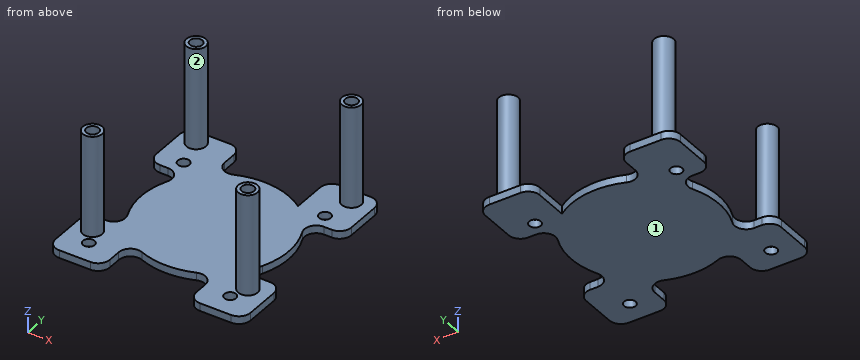
Autodesk Inventor part; units mm, degrees
ref_plane "Work Plane1" through (0, 0, 0) normal (0, 0, 1) x (1, 0, 0)
ref_plane "YZ Plane" through (0, 0, 0) normal (1, 0, 0) x (0, 1, 0)
ref_plane "XZ Plane" through (0, 0, 0) normal (0, 1, 0) x (-1, 0, 0)
ref_plane "Work Plane1" through (0, 0, 0) normal (0, 0, 1) x (1, 0, 0)
sketch "Sketch1" plane through (0, 0, 0) normal (0, 0, 1) x (1, 0, 0)
  circle A0 centre (22.2, -27.45) radius 1.5
  circle A1 centre (58.6, -27.45) radius 1.5
  circle A2 centre (22.2, 9.15) radius 1.5
  circle A3 centre (58.6, 9.15) radius 1.5
  line L0 (15.5, 16.5) -> (15.5, -25.3)
  line L1 (19.5, -29.3) -> (61, -29.3)
  line L2 (61, 20.5) -> (19.5, 20.5)
  line L3 (64.8607, 14) -> (64.8607, -18)
  line L4 (65.75, -18) -> (65.75, 14)
  line L5 (65.75, -33.3) -> (51.75, -33.3)
  line L6 (51.75, -33.3) -> (51.75, -21.8024)
  line L7 (55.4368, -18.3) -> (65.75, -18.3)
  line L8 (65.75, -18.3) -> (65.75, -33.3)
  line L9 (15.5, -33.3) -> (29.5, -33.3)
  line L10 (29.5, -33.3) -> (29.5, -21.8024)
  line L11 (25.8132, -18.3) -> (15.5, -18.3)
  line L12 (15.5, -18.3) -> (15.5, -33.3)
  line L13 (15.5, 20.5697) -> (29.5, 20.5697)
  line L14 (29.5, 20.5697) -> (29.5, 9.0024)
  line L15 (25.8695, 5.5697) -> (15.5, 5.5697)
  line L16 (15.5, 5.5697) -> (15.5, 20.5697)
  line L17 (51.75, 20.5697) -> (65.75, 20.5697)
  line L18 (65.75, 20.5697) -> (65.75, 5.5697)
  line L19 (65.75, 5.5697) -> (55.3805, 5.5697)
  line L20 (51.75, 9.0024) -> (51.75, 20.5697)
  arc A4 (51.75, 9.0024) -> (29.5, 9.0024) centre (40.625, -6.4) ccw
  arc A5 (25.8695, 5.5697) -> (25.8132, -18.3) centre (40.625, -6.4) ccw
  arc A6 (29.5, -21.8024) -> (51.75, -21.8024) centre (40.625, -6.4) ccw
  arc A7 (55.4368, -18.3) -> (55.3805, 5.5697) centre (40.625, -6.4) ccw
  line L21 (65.75, 20.5697) -> (65.75, 5.5697)
  line L22 (65.75, -18.3) -> (65.75, -33.3)
  line L23 (15.5, 20.5697) -> (29.5, 20.5697)
  line L24 (51.75, 20.5697) -> (65.75, 20.5697)
  line L25 (15.5, -33.3) -> (15.5, -18.3)
  line L26 (15.5, 5.5697) -> (15.5, 20.5697)
  point P0 (0, 0)
  point P1 (40.25, 20.5)
  dimension "d10" = 50.25
  dimension "d13" = 26.9
extrude "Extrusion1" add sketch "Sketch1" along normal blind 2 contours L16 L13 L14 A4 L20 L17 L18 L4 L19 A7 L7 L8 L5 L6 A6 L10 L9 L12 L0 L11 A5 L15
fillet "Fillet1" radius 3 7 edges at (55.3805, 5.5697, 1) (29.5, -21.8024, 1) (25.8132, -18.3, 1) (29.5, 9.0024, 1) (55.4368, -18.3, 1) (25.8695, 5.5697, 1) (51.75, -21.8024, 1)
fillet "Fillet2" radius 3 12 edges at (15.5, 20.5697, 1) (15.5, 5.5697, 1) (29.5, 20.5697, 1) (51.75, 20.5697, 1) (65.75, 20.5697, 1) (65.75, -18.3, 1) (51.75, -33.3, 1) (15.5, -18.3, 1) (15.5, -33.3, 1) (29.5, -33.3, 1) (65.75, -33.3, 1) (65.75, 5.5697, 1)
sketch "Sketch2" plane through (0, 0, 2) normal (0, 0, 1) x (1, 0, 0)
  circle A0 centre (60.25, -23.1) radius 1.6
  circle A1 centre (20.25, -23.1) radius 1.6
  circle A2 centre (20.25, 16.9) radius 1.6
  circle A3 centre (60.25, 16.9) radius 1.6
  circle A4 centre (20.25, -23.1) radius 2.5
  circle A5 centre (60.25, 16.9) radius 2.5
  circle A6 centre (20.25, 16.9) radius 2.5
  circle A7 centre (60.25, -23.1) radius 2.5
  point P0 (0, 0)
  dimension "d17" = 5
  dimension "d18" = 5
  dimension "d19" = 5
  dimension "d20" = 5
extrude "Extrusion2" add sketch "Sketch2" along normal blind 26
equation "\"d13\" = 0.5 * d11"
properties part number "soporteHBridge"
Verification items for the finished model (mm, model axes). Face numbers are marked on the shaded views. Coordinates: 2 decimals unless noted, no trailing zeros. Loops run counter-clockwise (first coordinate to the right, second up) from the corner with the lowest first, then second, coordinate; pieces in that order, holes last. Notation, with made-up numbers: (-26, 61) -> (24, 61) arc R12 ccw to (24, 74) -> close; hole circle Ø7 at (3, -40). An arc over 180 degrees is marked (long way). Answer as CSV lines item,"result".
1) Cross-section at B-B, the plane y = 16.9. Record the cut outline in (x, z).
Found:
outline,"(15.5, 0) -> (29.5, 0) -> (29.5, 2) -> (22.75, 2) -> (22.75, 28) -> (21.85, 28) -> (21.85, 2) -> (18.65, 2) -> (18.65, 28) -> (17.75, 28) -> (17.75, 2) -> (15.5, 2) -> close; (51.75, 0) -> (65.75, 0) -> (65.75, 2) -> (62.75, 2) -> (62.75, 28) -> (61.85, 28) -> (61.85, 2) -> (58.65, 2) -> (58.65, 28) -> (57.75, 28) -> (57.75, 2) -> (51.75, 2) -> close"
2) Cross-section at A-A, the plane z = 20.5. Record the cut outline in (x, y), then the cut area to 3 significant figures.
Found:
outline,"circle Ø5 at (20.25, -23.1); circle Ø5 at (20.25, 16.9); circle Ø5 at (60.25, -23.1); circle Ø5 at (60.25, 16.9); hole circle Ø3.2 at (20.25, -23.1); hole circle Ø3.2 at (20.25, 16.9); hole circle Ø3.2 at (60.25, -23.1); hole circle Ø3.2 at (60.25, 16.9)"
area,"46.4 mm2"
3) Depth check by flat-ended pin: pin 1 (3 mm diameter, centred on y = -21.5, z = 11, fed in from -X); pin 2 (3.5 mm diameter, centred on x = 60.25, y = 16.9, fed in from +Z); pin 3 (1.8 mm diameter, centred on x = 58.6, y = 9.15, fed in from -Z); pin 4 (12 mm diameter, centred on x = 22.5, y = 7.5, fed in from +Z). Enter the tip coordinate at first touch or a pass-through.
Found:
pin 1,"stops at x = 17.75"
pin 2,"stops at z = 28"
pin 3,"passes through"
pin 4,"stops at z = 2"
4) Cross-section at C-C, the plane x = 36.5. Record the cut outline in (y, z), then the cut area to 3 significant figures.
Found:
outline,"(-24.95, 0) -> (12.15, 0) -> (12.15, 2) -> (-24.95, 2) -> close"
area,"74.2 mm2"
5) Release check for a two-part mould opening along Y. For the marked faces 1 and 2 record: +Y half, -Y half, draft (parallel to the pull), parting line (faces both ways), or undercut.
Found:
face 1,"draft"
face 2,"undercut"
6) Cross-section at D-D, the plane y = -7.5. Record the cut outline in (x, z).
Found:
outline,"(21.66, 0) -> (59.59, 0) -> (59.59, 2) -> (21.66, 2) -> close"
7) Thickness scan on L1, parallel to Y at x = 20.25, z = 15.75; L2, parallel to X at y = 18, z = 16.25 (3 decimals); L3, parallel to X at y = 15.5, z = 26.5. Record the ranges inside material, lowest first. Write a range as from..to.
Found:
L1,"y = -25.6..-24.7, -21.5..-20.6, 14.4..15.3, 18.5..19.4"
L2,"x = 18.005..19.088, 21.412..22.495, 58.005..59.088, 61.412..62.495"
L3,"x = 18.18..19.48, 21.02..22.32, 58.18..59.48, 61.02..62.32"
